Part model, mm, in its own coordinate system. A direction names the side the tool comes from. Round coordinates to 2 decimals unless told otherwise and drop trailing zeros. Write each loop counter-clockwise with the first axis right and the second up, starting at its lowest first coordinate (ties: lowest second). Pieces come first, ordered by that corner, then holes. Notation, with made-up numbers: M 32,-18 L 67,-18 A16 ccw 67,9 Z; hole C -28,32 d8. An arc over 180 degrees is marked long. Answer as a JSON object with one key per item and string values. Group by question number.
1. Drill centre lines: line 1 (X direction, y = 1.7, z = 0); line 2 (Z direction, x = -0.5, y = 1.3); line 3 (X direction, y = 2.5, z = -45.5). Where is each one in solid material? Low to high. Write a range as from..to.
2. Band-saw the part on C-C, the plane z = -85. Write the cut outline in (x, y) (3 decimals), plus the area to 3 significant figures.
3. Two-plate mould, pull along Z, no slides. Class faces 3 (the face through (134.69, 1.57, 134.19)), 4 (the face through (-133, 3.175, -2)), 5 (the face through (98.267, 1.565, -98.77)): +Z half, -Z half, draft (parallel to the pull), parting line (faces both ways), or undercut.
4. Band-saw the part on A-A, the plane z = 20.5. Write the cut outline in (x, y) (3 decimals), plus the area to 3 significant figures.
5. Band-saw the part on B-B, the plane y = 2.2. Count the separate pieces of the cut face and the enclosed holes in it, plus the area to 3 significant figures.
6. Which spindle directions (+Z, -Z, +X, -X, +Y, -Y) get a long thin tool onto all of the face, cutting with end or side? Do faces 1 (the face through (134.19, 1.57, -134.69)), 2 (the face through (-123.687, 1.565, 78.869)). Say none if no direction does.
7. Drop a flat-ended pin along its axis: pin 1 (3.5 mm diameter, centred on x = 140.97, z = 0, fed in from -Y). Give the stop position or say it passes through.
from build123d import *

# Parameters (mm, degrees)
BOSS_EXTRUDE1_DEPTH = 3.175
SKETCH4_R           = 2.159
CUT_EXTRUDE2_DEPTH  = 216.549531721


with BuildPart() as part:
    # Sketch2 → Boss-Extrude1 (new body)
    with BuildSketch(Plane(origin=(0, 0, 0), x_dir=(1, 0, 0), z_dir=(0, 1, 0))):
        Polygon((-152.4, 116.478975516), (-116.478975516, 152.4), (116.478975516, 152.4), (152.4, 116.478975516), (152.4, -116.478975516), (116.478975516, -152.4), (-116.478975516, -152.4), (-152.4, -116.478975516), align=None)
        with BuildLine():
            Line((-116.478975516, 80.557951031), (-80.557951031, 116.478975516))
            ThreePointArc((-80.557951031, 116.478975516), (-78.800891411, 123.772159882), (-72.028975516, 127))
            Line((-72.028975516, 127), (-59.328975516, 127))
            Line((-59.328975516, 127), (59.328975516, 127))
            Line((59.328975516, 127), (72.028975516, 127))
            ThreePointArc((72.028975516, 127), (78.800891411, 123.772159882), (80.557951031, 116.478975516))
            Line((80.557951031, 116.478975516), (116.478975516, 80.557951031))
            ThreePointArc((116.478975516, 80.557951031), (123.772159882, 78.800891411), (127, 72.028975516))
            Line((127, 72.028975516), (127, 59.328975516))
            Line((127, 59.328975516), (127, -59.328975516))
            Line((127, -59.328975516), (127, -72.028975516))
            ThreePointArc((127, -72.028975516), (123.772159882, -78.800891411), (116.478975516, -80.557951031))
            Line((116.478975516, -80.557951031), (80.557951031, -116.478975516))
            ThreePointArc((80.557951031, -116.478975516), (78.800891411, -123.772159882), (72.028975516, -127))
            Line((72.028975516, -127), (59.328975516, -127))
            Line((59.328975516, -127), (-59.328975516, -127))
            Line((-59.328975516, -127), (-72.028975516, -127))
            ThreePointArc((-72.028975516, -127), (-78.800891411, -123.772159882), (-80.557951031, -116.478975516))
            Line((-80.557951031, -116.478975516), (-116.478975516, -80.557951031))
            ThreePointArc((-116.478975516, -80.557951031), (-123.772159882, -78.800891411), (-127, -72.028975516))
            Line((-127, -72.028975516), (-127, -59.328975516))
            Line((-127, -59.328975516), (-127, 59.328975516))
            Line((-127, 59.328975516), (-127, 72.028975516))
            ThreePointArc((-127, 72.028975516), (-123.772159882, 78.800891411), (-116.478975516, 80.557951031))
        make_face(mode=Mode.SUBTRACT)
    extrude(amount=BOSS_EXTRUDE1_DEPTH)

    # Sketch4 → Cut-Extrude2 (cut, through all)
    with BuildSketch(Plane(origin=(0, 3.175, 0), x_dir=(1, 0, 0), z_dir=(0, 1, 0))):
        with Locations(Location((0, 140.97, 0), (0, 0, 270))):
            Circle(SKETCH4_R)
        with Locations(Location((-50.8, 140.97, 0), (0, 0, 270))):
            Circle(SKETCH4_R)
        with Locations(Location((-140.97, 50.8, 0), (0, 0, 270))):
            Circle(SKETCH4_R)
        with Locations(Location((-140.97, 0, 0), (0, 0, 270))):
            Circle(SKETCH4_R)
        with Locations(Location((140.97, 0, 0), (0, 0, 90))):
            Circle(SKETCH4_R)
        with Locations(Location((140.97, 50.8, 0), (0, 0, 90))):
            Circle(SKETCH4_R)
        with Locations(Location((50.8, 140.97, 0), (0, 0, 90))):
            Circle(SKETCH4_R)
        with Locations(Location((50.8, -140.97, 0), (0, 0, 270))):
            Circle(SKETCH4_R)
        with Locations(Location((140.97, -50.8, 0), (0, 0, 270))):
            Circle(SKETCH4_R)
        with Locations(Location((-50.8, -140.97, 0), (0, 0, 90))):
            Circle(SKETCH4_R)
        with Locations(Location((0, -140.97, 0), (0, 0, 90))):
            Circle(SKETCH4_R)
        with Locations(Location((-140.97, -50.8, 0), (0, 0, 90))):
            Circle(SKETCH4_R)
    extrude(amount=-CUT_EXTRUDE2_DEPTH, mode=Mode.SUBTRACT)


solid = part.part
Worked answers:
{
 "1": {"line 1": "x = -152.4..-143.13, -138.81..-127, 127..138.81, 143.13..152.4", "line 2": "z = -152.4..-143.07, -138.87..-127, 127..138.87, 143.07..152.4", "line 3": "x = -152.4..-127, 127..152.4"},
 "2": {"outline": "M -152.4,0 L -112.037,0 L -112.037,3.175 L -152.4,3.175 Z; M 112.037,0 L 152.4,0 L 152.4,3.175 L 112.037,3.175 Z", "area": "256 mm^2"},
 "3": {"face 3": "+Z half", "face 4": "draft", "face 5": "undercut"},
 "4": {"outline": "M -152.4,0 L -127,0 L -127,3.175 L -152.4,3.175 Z; M 127,0 L 152.4,0 L 152.4,3.175 L 127,3.175 Z", "area": "161 mm^2"},
 "5": {"separate pieces": "1", "enclosed holes": "13", "area": "31,800 mm^2"},
 "6": {"face 1": "-Z, +X, +Y, -Y", "face 2": "+Y, -Y"},
 "7": {"pin 1": "passes through"}
}
